```python
from build123d import *

# Parameters (mm, degrees)
SKETCH3_W               = 1530.35
SKETCH3_H               = 44.45
BASE_FLANGE1_DEPTH      = 3.2639
EDGE_FLANGE1_DEPTH      = 1530.35
F_1_4_CLEARANCE_HOLE1_D = 6.7564
FILLET1_R               = 3.175


# Sheet-metal steps are written as plain solids
with BuildPart() as part:
    # Sketch3 → Base-Flange1 (new body)
    with BuildSketch(Plane(origin=(0, 0, 0), x_dir=(1, 0, 0), z_dir=(0, 1, 0))):
        with Locations((765.175, 22.225)):
            Rectangle(SKETCH3_W, SKETCH3_H)
    extrude(amount=-BASE_FLANGE1_DEPTH)

    # Edge-Flange1 section (across the edge) → Edge-Flange1 (add)
    with BuildSketch(Plane(origin=(0, -3.2639, -47.625), x_dir=(0, 0, 1), z_dir=(1, 0, 0))):
        with BuildLine():
            Line((-3.2639, 3.175), (-3.2639, 41.1861))
            Line((-3.2639, 41.1861), (0, 41.1861))
            Line((0, 41.1861), (0, 3.175))
            ThreePointArc((0, 3.175), (0.92993597, 0.92993597), (3.175, 0))
            Line((3.175, 0), (3.175, -3.2639))
            ThreePointArc((3.175, -3.2639), (-1.377989853, -1.377989853), (-3.2639, 3.175))
        make_face()
    extrude(amount=EDGE_FLANGE1_DEPTH)

    # 1/4 Clearance Hole1 (through all)
    with Locations(Plane(origin=(0, 0, 0), x_dir=(1, 0, 0), z_dir=(0, 1, 0))):
        with Locations((22.225, 22.225), (1508.125, 22.225)):
            Hole(F_1_4_CLEARANCE_HOLE1_D / 2)

    # Fillet1
    fillet1_edges = [part.edges().sort_by_distance(p)[0] for p in [
        (0, -44.45, -49.25695),
        (1530.35, -44.45, -49.25695),
        (1530.35, -1.63195, 0),
        (0, -1.63195, 0),
    ]]
    fillet(fillet1_edges, radius=FILLET1_R)


solid = part.part
```
Verification items for the finished model (mm, model axes). A direction names the side the tool comes from. Give positions to 0.01 mm unless a question says otherwise; leave off trailing zeros. Order: outer loops, then holes, each group sorted by start corner. A loop starts at its lowest first (then second) coordinate and runs counter-clockwise, first axis right, second up. Notation, with made-up numbers: M -37.5,4 L 5.5,4 A22 ccw 5.5,15 Z; hole C 69,34 d3. An arc over 180 degrees is marked long. Answer in a Markdown table with one row per item. Add a question column.
Item 1: Section check B-B, the plane y = -32. Enter the section's corners in (x, z) (3 decimals).
Item 2: Tool access check on faces 1 (the flat face through (754, 0, -23)), 2 (the flat face through (754, -3.264, -23)). Record the directions out of +Z, -Z, +X, -X, +Y, -Y that give a thin tool (end or side, any length) a straight path to the whole face; none if there is none.
Item 3: Section check A-A, the plane x = 333. Enter the section's corners in (y, z) (3 decimals).
Item 4: Section check C-C, the plane z = -35. Enter the section's corners in (x, y).
Item 5: Gauge pin test, flat ends, axial feed: pin 1 (11.5 mm diameter, centred on x = 868, y = -21, fed in from +Z) (3 decimals); pin 2 (1.5 mm diameter, centred on x = 826.5, z = -32, fed in from -Y); pin 3 (11 mm diameter, centred on x = 22.225, z = -22.225, fed in from +Y); pin 4 (8 mm diameter, centred on x = 343.5, y = -8.5, fed in from +Z). Record the tip position at first contact, or that the pin passes through.
Item 6: Scan lines: probe 1 along Y at (x, z) = (1392.5, -18.5); probe 2 along Z at (x, y) = (511.5, -35.5) (3 decimals); probe 3 along Z at (x, y) = (709.5, -3). Record each from-to range of solid material in increasing order. Write a range as from..to.
Filled sheet:
| question | item | result |
|---|---|---|
| 1 | outline | M 0,-50.889 L 1530.35,-50.889 L 1530.35,-47.625 L 0,-47.625 Z |
| 2 | face 1 | +Z, -Z, +X, -X, +Y |
| 2 | face 2 | +Z, +X, -X, -Y |
| 3 | outline | M -44.45,-50.889 L -6.439,-50.889 A6.439 ccw 0,-44.45 L 0,0 L -3.264,0 L -3.264,-44.45 A3.175 cw -6.439,-47.625 L -44.45,-47.625 Z |
| 4 | outline | M 0,-3.26 L 1530.35,-3.26 L 1530.35,0 L 0,0 Z |
| 5 | pin 1 | stops at z = -47.625 |
| 5 | pin 2 | stops at y = -3.26 |
| 5 | pin 3 | stops at y = 0 |
| 5 | pin 4 | stops at z = -46.96 |
| 6 | probe 1 | y = -3.26..0 |
| 6 | probe 2 | z = -50.889..-47.625 |
| 6 | probe 3 | z = -49.89..0 |
